from build123d import *

# Parameters (mm, degrees)
SKETCH_1_R          = 1.5
SKETCH_1_R_2        = 4.05
EXTRUDE_1_DEPTH     = 2
SKETCH_2_R          = 0.5
CUT_EXTRUDE_1_DEPTH = 10
FILLET_1_R          = 1


with BuildPart() as part:
    # 草图1 → 凸台-拉伸1 (new body)
    with BuildSketch(Plane.XY):
        Polygon((-5, -43.5), (5, -43.5), (5, -23.6), (-5.1, -23.6), (-5.1, -13.4), (5, -13.4), (5, 7.5), (-47, 7.5), (-47, -7.4), (-34.9, -7.4), (-34.9, -13.6), (-47, -13.6), (-47, -14.091283395), align=None)
        with Locations((-32, 0)):
            Circle(SKETCH_1_R, mode=Mode.SUBTRACT)
        Circle(SKETCH_1_R, mode=Mode.SUBTRACT)
        with Locations((0, -38.5)):
            Circle(SKETCH_1_R, mode=Mode.SUBTRACT)
        with Locations((0, -28.5)):
            Circle(SKETCH_1_R, mode=Mode.SUBTRACT)
        with Locations((-20, 0)):
            Circle(SKETCH_1_R_2, mode=Mode.SUBTRACT)
    extrude(amount=EXTRUDE_1_DEPTH)

    # 草图2 → 切除-拉伸1 (cut)
    with BuildSketch(Plane.XY.offset(2)):
        with Locations((-34.9, -7.4)):
            Circle(SKETCH_2_R)
        with Locations((-34.9, -13.6)):
            Circle(SKETCH_2_R)
        with Locations((-5.1, -13.4)):
            Circle(SKETCH_2_R)
        with Locations((-5.1, -23.6)):
            Circle(SKETCH_2_R)
    extrude(amount=-CUT_EXTRUDE_1_DEPTH, mode=Mode.SUBTRACT)

    # 圆角1
    fillet_1_edges = [part.edges().sort_by_distance(p)[0] for p in [
        (-47, -7.4, 1),
        (-47, 7.5, 1),
        (5, 7.5, 1),
        (5, -13.4, 1),
        (5, -23.6, 1),
        (5, -43.5, 1),
        (-5, -43.5, 1),
    ]]
    fillet(fillet_1_edges, radius=FILLET_1_R)


solid = part.part
For this review, take the finished solid that the model builds, in its own axes (mm). A direction names the side the tool comes from. Round coordinates to 2 decimals unless told otherwise and drop trailing zeros. Loops run counter-clockwise (first coordinate to the right, second up) from the corner with the lowest first, then second, coordinate; pieces in that order, holes last. Notation, with made-up numbers: (86.25, -19.5) - (141.25, -19.5) arc R22 cw to (141.25, 12.5) - close; hole circle Ø3 at (55.5, 85.25). An arc over 180 degrees is marked (long way). One line per item, written item: value. Start each with the question number.
Item 1: Take a section at B-B (z = 1.25). State how many separate pieces and enclosed holes the cut face has, plus the area to 3 significant figures.
Item 2: Take a section at C-C (y = -38.5). Give the boundary of the cut face in (x, z).
Item 3: For faces 5 (the flat face through (-5.1, -19, 1)), 6 (the flat face through (-34.9, -10, 1)), 7 (the flat face through (-16, -12, 2)), list the 3-axis set-ups (+Z, -Z, +X, -X, +Y, -Y) from which the entire face can be reached by the end or side of a thin tool; tool diameter is ignored.
Item 4: The part is to be moulded in two halves that separate along Y. For faces 1 (the flat face through (0, -13.4, 1)), 2 (the flat face through (5, -34, 1)), 3 (the flat face through (0, -43.5, 1)), 4 (the cylindrical face through (-1.5, 0.07, 0.99)), say which applies: +Y half, -Y half, draft (parallel to the pull), parting line (faces both ways), or undercut.
Item 5: For L1, parallel to Y at x = 0, z = 1.55; L2, parallel to Y at x = 1, z = 0.95; L3, parallel to Y at x = -4, z = 1.7, list the stretches that pass through material, from the lowest coordinate up.
Item 6: Clearance check with flat-ended pins moving along their axes: pin 1 Ø1.8 at (x, y) = (0, 0) entering from -Z; pin 2 Ø1.5 at (x, y) = (-23, -16.5) entering from -Z; pin 3 Ø0.6 at (y, z) = (-10, 1) entering from -X. State where each tip first meets the part, or that it passes through.
Item 7: Take a section at A-A (x = 0). Give the boundary of the cut face in (y, z).
Item 8: Take a section at D-D (x = -20). Give the boundary of the cut face in (y, z), plus the area to 3 significant figures.
Answer below:
1. separate pieces: 1
1. enclosed holes: 5
1. area: 1,770 mm2
2. outline: (-12.14, 0) - (-1.5, 0) - (-1.5, 2) - (-12.14, 2) - close; (1.5, 0) - (5, 0) - (5, 2) - (1.5, 2) - close
3. face 5: +Z, -Z, +X
3. face 6: +Z, -Z, -X
3. face 7: +Z, +X, -X, +Y, -Y
4. face 1: undercut
4. face 2: draft
4. face 3: -Y half
4. face 4: undercut
5. L1: y = -43.5 to -40, -37 to -30, -27 to -23.6, -13.4 to -1.5, 1.5 to 7.5
5. L2: y = -43.5 to -39.62, -37.38 to -29.62, -27.38 to -23.6, -13.4 to -1.12, 1.12 to 7.5
5. L3: y = -43.5 to -23.6, -13.4 to 7.5
6. pin 1: passes through
6. pin 2: stops at z = 0
6. pin 3: stops at x = -34.9
7. outline: (-43.5, 0) - (-40, 0) - (-40, 2) - (-43.5, 2) - close; (-37, 0) - (-30, 0) - (-30, 2) - (-37, 2) - close; (-27, 0) - (-23.6, 0) - (-23.6, 2) - (-27, 2) - close; (-13.4, 0) - (-1.5, 0) - (-1.5, 2) - (-13.4, 2) - close; (1.5, 0) - (7.5, 0) - (7.5, 2) - (1.5, 2) - close
8. outline: (-33, 0) - (-4.05, 0) - (-4.05, 2) - (-33, 2) - close; (4.05, 0) - (7.5, 0) - (7.5, 2) - (4.05, 2) - close
8. area: 64.8 mm2
